from build123d import *

# Parameters (mm, degrees)
SKETCH6_W           = 220
SKETCH6_H           = 175
SKETCH6_R           = 11
SKETCH6_R_2         = 24
BOSS_EXTRUDE1_DEPTH = 6.75


with BuildPart() as part:
    # Sketch6 → Boss-Extrude1 (new body)
    # profile 1 of 2: a face of its own
    with BuildSketch(Plane.XY):
        with Locations((-459.776309557, -210.085944494)):
            Rectangle(SKETCH6_W, SKETCH6_H)
        with Locations((-459.807870528, -262.585944494)):
            Circle(SKETCH6_R, mode=Mode.SUBTRACT)
        with Locations((-407.846346301, -172.585944494)):
            Circle(SKETCH6_R, mode=Mode.SUBTRACT)
        with Locations((-511.769394755, -172.585944494)):
            Circle(SKETCH6_R, mode=Mode.SUBTRACT)
        with Locations((-459.807870528, -202.585944494)):
            Circle(SKETCH6_R_2, mode=Mode.SUBTRACT)
    # profile 2 of 2: a face of its own
    with BuildSketch(Plane.XY):
        with Locations((-459.807870528, -202.585944494)):
            Circle(SKETCH6_R_2)
    extrude(amount=BOSS_EXTRUDE1_DEPTH)


solid = part.part
Here's how the part is built. I have some questions about the finished solid (model axes, mm). Round coordinates to 2 decimals unless told otherwise and drop trailing zeros. Loops run counter-clockwise (first coordinate to the right, second up) from the corner with the lowest first, then second, coordinate; pieces in that order, holes last. Notation, with made-up numbers: (25.5, 12.25) -> (38.5, 12.25) arc R28 cw to (38.5, 40.25) -> close; hole circle Ø1 at (82.25, 60.25). An arc over 180 degrees is marked (long way). Write each question's results on one line, items separated by ' | '.
(1) If we section it at B-B, the plane y = -176: List the corners of the cut face in (x, z) for me.
Worked answers:
outline: (-569.78, 0) -> (-522.23, 0) -> (-522.23, 6.75) -> (-569.78, 6.75) -> close; (-501.31, 0) -> (-418.3, 0) -> (-418.3, 6.75) -> (-501.31, 6.75) -> close; (-397.39, 0) -> (-349.78, 0) -> (-349.78, 6.75) -> (-397.39, 6.75) -> close
(2) For P1, Ø13, axis at x = -511.77, y = -172.59, coming from the -Z side, with a flat end and sliding along its axis, tell me the tip position at first contact or that it passes through.
Worked answers:
P1: through
(3) We'd pull the mould along Y, two halves only. Please class faces 1 (the face through (-449.647, -266.799, 3.328)), 2 (the face through (-349.776, -211, 3)), 3 (the face through (-461, -122.586, 3)): released by +Y, released by -Y, zero draft, split by the parting line, or undercut.
Worked answers:
face 1: undercut | face 2: zero draft | face 3: released by +Y
(4) If we section it at A-A, the plane x = -505.5: List the corners of the cut face in (y, z) for me.
Worked answers:
outline: (-297.59, 0) -> (-181.62, 0) -> (-181.62, 6.75) -> (-297.59, 6.75) -> close; (-163.55, 0) -> (-122.59, 0) -> (-122.59, 6.75) -> (-163.55, 6.75) -> close
(5) If I drill on L1, parallel to Y at x = -511, z = 3.75; L2, parallel to X at y = -168, z = 1; L3, parallel to Y at x = -405.5, z = 5.75, over which ranges is the centre line in solid material (lowest first)?
Worked answers:
L1: -297.59 to -183.56, -161.61 to -122.59 | L2: -569.78 to -521.77, -501.77 to -417.84, -397.85 to -349.78 | L3: -297.59 to -183.33, -161.84 to -122.59
(6) If we section it at C-C, the plane z = 1.5: List the corners of the cut face in (x, y) for me.
Worked answers:
outline: (-569.78, -297.59) -> (-349.78, -297.59) -> (-349.78, -122.59) -> (-569.78, -122.59) -> close; hole circle Ø22 at (-511.77, -172.59); hole circle Ø22 at (-459.81, -262.59); hole circle Ø22 at (-407.85, -172.59)
